The listing builds one solid part. Answer for the finished solid, in the listing's coordinates (mm). A direction names the side the tool comes from. Round coordinates to 2 decimals unless told otherwise and drop trailing zeros. Write each loop counter-clockwise with the first axis right and the second up, starting at its lowest first coordinate (ties: lowest second). Pieces come first, ordered by that corner, then holes. Notation, with made-up numbers: (42, 21) - (60, 21) arc R13 cw to (60, 43) - close; hole circle Ø1 at (13.5, 19). An arc over 180 degrees is marked (long way). Answer in a Markdown table with one row per item.
from build123d import *

# Parameters (mm, degrees)
SKETCH_1_W          = 175
SKETCH_1_H          = 63
EXTRUDE_1_DEPTH     = 5
CUT_EXTRUDE_1_REACH = 106.006
CHAMFER_1_SIZE      = 15
CHAMFER_2_SIZE      = 5


with BuildPart() as part:
    # 草图1 → 凸台-拉伸1 (new body)
    with BuildSketch(Plane.XY):
        with Locations((0, 24.5)):
            Rectangle(SKETCH_1_W, SKETCH_1_H)
    extrude(amount=EXTRUDE_1_DEPTH)

    # 草图2 → 切除-拉伸1 (cut, up to next)
    with BuildSketch(Plane.XY.offset(5), mode=Mode.PRIVATE) as cut_extrude_1_sk1:
        Polygon((-74.5, 56), (-4.5, 56), (-4.5, 43.378679656), (-10.378679656, 37.5), (-68.621320344, 37.5), (-74.5, 43.378679656), align=None)
    cut_extrude_1_tool1 = extrude(cut_extrude_1_sk1.sketch, amount=-CUT_EXTRUDE_1_REACH, mode=Mode.PRIVATE) & part.part
    add(cut_extrude_1_tool1.solids().sort_by_distance((-39.5, 46.94989, 5))[0], mode=Mode.SUBTRACT)

    # 倒角1
    chamfer_1_edges = [part.edges().sort_by_distance(p)[0] for p in [
        (87.5, -7, 2.5),
        (-87.5, -7, 2.5),
    ]]
    chamfer(chamfer_1_edges, length=CHAMFER_1_SIZE)

    # 倒角2
    chamfer_2_edges = [part.edges().sort_by_distance(p)[0] for p in [
        (-87.5, 56, 2.5),
        (87.5, 56, 2.5),
    ]]
    chamfer(chamfer_2_edges, length=CHAMFER_2_SIZE)


solid = part.part
(1) Find the intervals of material crossed by line 1 (X direction, y = 46, z = 0.35); line 2 (Y direction, x = -56, z = 0.5); line 3 (X direction, y = 0, z = 3.35), in increasing order.
Checked values:
| item | result |
|---|---|
| line 1 | x = -87.5 to -74.5, -4.5 to 87.5 |
| line 2 | y = -7 to 37.5 |
| line 3 | x = -79.5 to 79.5 |
(2) Section B-B (x = -38.5) is taken. Give the vertices of the cut face in (y, z).
Checked values:
| item | result |
|---|---|
| outline | (-7, 0) - (37.5, 0) - (37.5, 5) - (-7, 5) - close |
(3) A flat-ended cylindrical pin translates along its axis: pin 1 (5 mm diameter, centred on x = -60, y = 17, fed in from -Z). Find the tip coordinate at first contact, or state that the pin passes through.
Checked values:
| item | result |
|---|---|
| pin 1 | stops at z = 0 |
(4) For a pull along X with two mould halves and no side action, classify faces 3 (the flat face through (-85, 53.5, 2.5)), 4 (the flat face through (-39, 37.5, 3)), 5 (the flat face through (38, 56, 2)) as pulls with the +X half, pulls with the -X half, needs draft (parallel to the pull), parting line crosses it, or undercut.
Checked values:
| item | result |
|---|---|
| face 3 | pulls with the -X half |
| face 4 | undercut |
| face 5 | needs draft |
(5) For faces 1 (the flat face through (-4.5, 50, 3)), 2 (the flat face through (-1, -7, 2)), determine the directions among +Z, -Z, +X, -X, +Y, -Y from which every point of the face is accessible in a straight line to the end or side of a thin tool.
Checked values:
| item | result |
|---|---|
| face 1 | +Z, -Z, +Y |
| face 2 | +Z, -Z, +X, -X, -Y |
(6) Section A-A (z = 0.85) is taken. Give the vertices of the cut face in (x, y).
Checked values:
| item | result |
|---|---|
| outline | (-87.5, 8) - (-72.5, -7) - (72.5, -7) - (87.5, 8) - (87.5, 51) - (82.5, 56) - (-4.5, 56) - (-4.5, 43.38) - (-10.38, 37.5) - (-68.62, 37.5) - (-74.5, 43.38) - (-74.5, 56) - (-82.5, 56) - (-87.5, 51) - close |
